The model under review builds one solid part; all positions refer to its coordinate system, in mm. Round coordinates to 2 decimals unless told otherwise and drop trailing zeros. Order: outer loops, then holes, each group sorted by start corner. A loop starts at its lowest first (then second) coordinate and runs counter-clockwise, first axis right, second up. Notation, with made-up numbers: M 67,-1 L 111,-1 A13 cw 111,5 Z; hole C 21,64 d5. An arc over 180 degrees is marked long. Answer as a JSON object with one key per item and string values. Group by question number.
1. Add section A-A on x = 0. State the section outline as (y, z) points, and give its area (3 significant figures).
2. Clearance check with flat-ended pins moving along their axes: P1, Ø4, axis at x = -42.5, z = -22, coming from the +Y side; P2, Ø2, axis at x = -32, y = 4.5, coming from the +Z side. State where each tip first meets the part, or that it passes through.
3. To check wall thickness, follow probe 1 along X at (y, z) = (2.45, -22); probe 2 along Z at (x, y) = (-43, 3.5); probe 3 along X at (y, z) = (1, -8.5). State the ranges of each line that lie inside material, in increasing order. Write a range as [from, to].
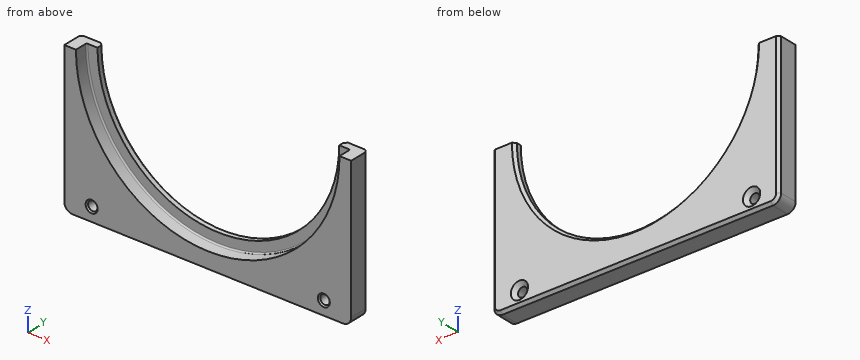
```python
from build123d import *

# Parameters (mm, degrees)
SKETCH1_W                                      = 105
SKETCH1_H                                      = 54
BOSS_EXTRUDE2_DEPTH                            = 7.5
SKETCH2_R                                      = 48.25
CUT_EXTRUDE1_DEPTH                             = 4.75
SKETCH3_R                                      = 44.25
CUT_EXTRUDE2_DEPTH                             = 60.510503275
CSK_FOR_M3_FLAT_HEAD_MACHINE_SCREW1_AT_2_COUNT = 2
CSK_FOR_M3_FLAT_HEAD_MACHINE_SCREW1_AT_2_PITCH = 85
FILLET1_R                                      = 3
CHAMFER1_SIZE                                  = 1
FILLET2_R                                      = 0.5


with BuildPart() as part:
    # Sketch1 → Boss-Extrude2 (new body)
    with BuildSketch(Plane(origin=(0, 0, 0), x_dir=(1, 0, 0), z_dir=(0, 1, 0))):
        Rectangle(SKETCH1_W, SKETCH1_H)
    extrude(amount=BOSS_EXTRUDE2_DEPTH)

    # Sketch2 → Cut-Extrude1 (cut)
    with BuildSketch(Plane.XZ):
        with Locations((0, 27)):
            Circle(SKETCH2_R)
    extrude(amount=-CUT_EXTRUDE1_DEPTH, mode=Mode.SUBTRACT)

    # Sketch3 → Cut-Extrude2 (cut, through all)
    with BuildSketch(Plane(origin=(0, 7.5, 0), x_dir=(1, 0, 0), z_dir=(0, 1, 0))):
        with Locations((0, -27)):
            Circle(SKETCH3_R)
    extrude(amount=-CUT_EXTRUDE2_DEPTH, mode=Mode.SUBTRACT)

    # Sketch5 → CSK for M3 Flat Head Machine Screw1 (revolve, cut)
    with BuildSketch(Plane(origin=(-42.5, 7.5, -22), x_dir=(0, 0, 1), z_dir=(1, 0, 0))):
        Polygon((0, 0), (0, 7.5), (2.2, 7.5), (1.7, 7), (1.7, 1.45), (3.15, 0), align=None)
    csk_for_m3_flat_head_machine_screw1 = revolve(axis=Axis((-42.5, 13.85, -22), (0, -1, 0)), mode=Mode.SUBTRACT)

    # CSK for M3 Flat Head Machine Screw1 at 2: CSK for M3 Flat Head Machine Screw1 ×2
    with Locations(*[(i * CSK_FOR_M3_FLAT_HEAD_MACHINE_SCREW1_AT_2_PITCH, 0, 0) for i in range(1, CSK_FOR_M3_FLAT_HEAD_MACHINE_SCREW1_AT_2_COUNT)]):
        add(csk_for_m3_flat_head_machine_screw1, mode=Mode.SUBTRACT)

    # Fillet1
    fillet1_edges = [part.edges().sort_by_distance(p)[0] for p in [
        (-52.5, 3.75, -27),
        (52.5, 3.75, -27),
    ]]
    fillet(fillet1_edges, radius=FILLET1_R)

    # Chamfer1
    chamfer1_edges = [part.edges().sort_by_distance(p)[0] for p in [
        (0, 7.5, -17.25),
        (52.5, 7.5, 1.5),
        (-52.5, 7.5, 1.5),
        (0, 7.5, -27),
        (51.621320344, 7.5, -26.121320344),
        (-51.621320344, 7.5, -26.121320344),
    ]]
    chamfer(chamfer1_edges, length=CHAMFER1_SIZE)

    # Fillet2
    fillet2_edges = [part.edges().sort_by_distance(p)[0] for p in [
        (0, 4.75, -21.25),
    ]]
    fillet(fillet2_edges, radius=FILLET2_R)


solid = part.part
```
Recorded:
{
 "1": {"outline": "M 0,-27 L 6.5,-27 L 7.5,-26 L 7.5,-18.25 L 6.5,-17.25 L 4.75,-17.25 L 4.75,-20.75 A0.5 cw 4.25,-21.25 L 0,-21.25 Z", "area": "53.2 mm²"},
 "2": {"P1": "stops at y = 6.35", "P2": "stops at z = -2.52"},
 "3": {"probe 1": "x = [-52.5, -44.2], [-40.8, 40.8], [44.2, 52.5]", "probe 2": "z = [-27, -23.62], [-20.38, 5.11]", "probe 3": "x = [-52.5, -32.68], [32.68, 52.5]"}
}
